Read the model definition and answer for the solid it produces. Units are mm, in the model's axes. A direction names the side the tool comes from. Coordinates: 2 decimals unless noted, no trailing zeros. Loops run counter-clockwise (first coordinate to the right, second up) from the corner with the lowest first, then second, coordinate; pieces in that order, holes last. Notation, with made-up numbers: (16, 65.25) -> (36, 65.25) arc R25 ccw to (36, 101.25) -> close; hole circle Ø2 at (49, -21). An arc over 180 degrees is marked (long way). Answer as a JSON object with one key per item and string values. Group by question number.
1) Consider probe 1 along Z at (x, y) = (11.5, -2.5); probe 2 along Z at (x, y) = (15.25, 0); probe 3 along Y at (x, z) = (27, 0). Determine where each line is inside the solid, lowest interval first. Write a range as [from, to].
2) Section A-A, the plane x = 12 is taken. Give the vertices of the cut face in (y, z), plus the area to 3 significant figures.
3) Determine the mould class of faces 1 (the face through (38.66, -5.72, -21.34)), 2 (the face through (36.714, -0.14, 5.712)), 3 (the face through (10.1, 10.6, 3.3)) for opening direction X: released by +X, released by -X, zero draft, split by the parting line, or undercut.
4) Which of the six approach directions +Z, -Z, +X, -X, +Y, -Y give full straight-line access (tool end or side, diameter ignored) to faces 4 (the face through (10.14, -2.038, -9.176)), 5 (the face through (23, 5, -31.2)), 6 (the face through (40.01, 6.755, -21.06))?
5) Section B-B, the plane z = -23 is taken. Give the vertices of the cut face in (x, y).
6) Flat-ended cylindrical pins translate along their axes: P1, Ø6, axis at x = 36, y = -1, coming from the -Z side; P2, Ø5, axis at x = 9, z = -2.5, coming from the +Y side; P3, Ø5, axis at x = 9.5, y = 9, coming from the +Z side. Find the tip coordinate at first contact, or state that the pin passes through.
Autodesk Inventor part; units mm, degrees
ref_plane "Work Plane2" through (21.213203, 0, 21.213203) normal (0.7071068, 0, 0.7071068) x (0, 1, 0)
ref_plane "XZ Plane" through (0, 0, 0) normal (0, 1, 0) x (-1, 0, 0)
ref_plane "XY Plane" through (0, 0, 0) normal (0, 0, 1) x (1, 0, 0)
sketch "Sketch1" plane through (0, 0, 0) normal (0, 0, 1) x (1, 0, 0)
  line L0 (0, 0) -> (0, 11) construction
  line L1 (0, 0) -> (20, 0) construction
  line L2 (20, 0) -> (20, 11.2) construction
  line L3 (0, 11) -> (20, 11.2)
  line L4 (0, 9.4) -> (20, 9.4)
  line L5 (20, 9.4) -> (20, 11.2)
  line L6 (0, 9.4) -> (0, 11)
  dimension "d0" = 11
  dimension "d1" = 20
  dimension "d2" = 11.2
  dimension "d3" = 1.6
sketch "Sketch1 outline for Revolution1" plane through (0, 0, 0) normal (0, 0, 1) x (1, 0, 0)
  line L0 (20, 9.4) -> (20, 11.2)
  line L1 (0, 9.4) -> (20, 9.4)
  line L2 (0, 11) -> (0, 9.4)
  line L3 (20, 11.2) -> (0, 11)
revolve "Revolution1" add sketch "Sketch1 outline for Revolution1" angle 360 about axis through (0, 0, 0) along (1, 0, 0)
sketch "Sketch2" plane through (20, 0, 0) normal (1, 0, 0) x (0, 0, -1)
  line L0 (0, 0) -> (11.2, 0) construction
  circle A0 centre (0, 0) radius 11.2 construction
  line L1 (11.2, 0) -> (11.2, 11.2) construction
  circle A1 centre (0, 0) radius 11.2
  circle A2 centre (0, 0) radius 9.4
  dimension "d5" = 11.2
sketch "Sketch2 outline for Revolution2" plane through (20, 0, 0) normal (1, 0, 0) x (0, 0, -1)
  circle A0 centre (0, 0) radius 11.2
  circle A1 centre (0, 0) radius 9.4
revolve "Revolution2" add sketch "Sketch2 outline for Revolution2" angle 90 about axis through (20, 0, -11.2) along (0, 1, 0)
sketch "Sketch3" plane through (0, 0, 0) normal (0, 1, 0) x (-1, 0, 0)
  line L0 (-42.4, -11.2) -> (-20, -11.2) construction
  line L1 (-31.2, -11.2) -> (-31.2, -31.2) construction
  line L2 (-31.2, -11.2) -> (-11.2, -11.2) construction
  line L3 (-31.2, -31.2) -> (-20.2, -31.2) construction
  line L4 (-20.2, -31.2) -> (-20, -11.2)
  line L5 (-20.2, -31.2) -> (-21.8, -31.2)
  line L6 (-21.8, -31.2) -> (-21.8, -11.2)
  line L7 (-20, -11.2) -> (-21.8, -11.2)
  point P0 (0, 0)
  dimension "d7" = 20
  dimension "d8" = 90
  dimension "d9" = 11
  dimension "d10" = 1.6
sketch "Sketch3 outline for Revolution3" plane through (0, 0, 0) normal (0, 1, 0) x (-1, 0, 0)
  line L0 (-20.2, -31.2) -> (-20, -11.2)
  line L1 (-21.8, -31.2) -> (-20.2, -31.2)
  line L2 (-21.8, -11.2) -> (-21.8, -31.2)
  line L3 (-20, -11.2) -> (-21.8, -11.2)
revolve "Revolution3" add sketch "Sketch3 outline for Revolution3" angle 360 about axis through (31.2, 0, -11.2) along (0, 0, -1)
ref_plane "Work Plane2" through (21.213203, 0, 21.213203) normal (0.7071068, 0, 0.7071068) x (0, 1, 0)
ref_plane "Work Plane1" through (0, 0, 0) normal (0.7071068, 0, 0.7071068) x (0, 1, 0)
sketch "Sketch4" plane through (21.213203, 0, 21.213203) normal (0.7071068, 0, 0.7071068) x (0, 1, 0)
  ellipse E0 centre (0, -14.142136) end of major axis (11.2, -14.142136) minor radius 7.919596 construction
  ellipse E1 centre (0, -29.981328) end of major axis (11.2, -29.981328) minor radius 7.919596 construction
  line L0 (0, -14.142136) -> (0, -29.981328) construction
  circle A0 centre (0, -22.061732) radius 10
  point P0 (0, 0)
  dimension "d14" = 20
sketch "Sketch4 outline for Extrusion1" plane through (21.213203, 0, 21.213203) normal (0.7071068, 0, 0.7071068) x (0, 1, 0)
  circle A0 centre (0, -22.061732) radius 10
extrude "Extrusion1" add sketch "Sketch4 outline for Extrusion1" against normal up to surface
equation "\"d0\" = 0.5 * TMStart"
equation "\"d1\" = TDepth"
equation "\"d2\" = 0.5 * TMEnd"
equation "\"d3\" = WallT"
equation "\"d5\" = BendR"
equation "\"d7\" = TDepth"
equation "\"d9\" = 0.5 * TMStart"
equation "\"d10\" = WallT"
equation "\"TMStart\" = 22"
equation "\"TMEnd\" = 22.4"
equation "\"WallT\" = 1.6"
equation "\"TDepth\" = 20"
equation "\"BendR\" = 0.5 * TMEnd"
properties part number "MtoM90degree"
Determined:
{
 "1": {"probe 1": "[-10.83, -9.06], [9.06, 10.83]", "probe 2": "[-11.15, -9.4], [9.4, 11.15]", "probe 3": "[-11.02, -9.18], [9.18, 11.02]"},
 "2": {"outline": "circle Ø22.24 at (0, 0); hole circle Ø18.8 at (0, 0)", "area": "111 mm²"},
 "3": {"face 1": "undercut", "face 2": "released by +X", "face 3": "released by -X"},
 "4": {"face 4": "-X", "face 5": "-Z, +X, -X, +Y, -Y", "face 6": "-Z"},
 "5": {"outline": "circle Ø22.16 at (31.2, 0); hole circle Ø18.8 at (31.2, 0)"},
 "6": {"P1": "z = -3.45", "P2": "y = 11.1", "P3": "z = 8.99"}
}
